from build123d import *

# Parameters (mm, degrees)
SKETCH1_R           = 2.15
SKETCH1_R_2         = 0.875
BOSS_EXTRUDE1_DEPTH = 12
SKETCH2_R           = 3
SKETCH2_R_2         = 0.874277104
BOSS_EXTRUDE2_DEPTH = 6.75
CUT_EXTRUDE1_DEPTH  = 14.5


with BuildPart() as part:
    # Sketch1 → Boss-Extrude1 (new body)
    with BuildSketch(Plane.XY):
        Circle(SKETCH1_R)
        Circle(SKETCH1_R_2, mode=Mode.SUBTRACT)
    extrude(amount=BOSS_EXTRUDE1_DEPTH)

    # Sketch2 → Boss-Extrude2 (add)
    with BuildSketch(Plane.XY.offset(12)):
        Circle(SKETCH2_R)
        Circle(SKETCH2_R_2, mode=Mode.SUBTRACT)
    extrude(amount=BOSS_EXTRUDE2_DEPTH)

    # Sketch3 → Cut-Revolve1 (revolve, cut)
    with BuildSketch(Plane(origin=(0, 0, 0), x_dir=(1, 0, 0), z_dir=(0, 1, 0))):
        Polygon((2.15, -12), (3, -13.75), (4.254862661, -13.125400589), (3.126580546, -11.371696522), align=None)
        Polygon((2.375, -18.75), (3, -15), (5.751760011, -16.421813113), (4.254862661, -20.939605223), align=None)
    revolve(axis=Axis((0, 0, 0), (0, 0, 1)), mode=Mode.SUBTRACT)

    # Sketch4 → Cut-Extrude1 (cut)
    with BuildSketch(Plane.XY.offset(18.75)):
        Polygon((0, 3.340763125), (-0.25, 3.340763125), (-0.25, 0.464842209), (0.25, 0.464842209), (0.25, 3.340763125), align=None)
        Polygon((3.340763125, 0), (3.340763125, 0.25), (0.464842209, 0.25), (0.464842209, -0.25), (3.340763125, -0.25), align=None)
        Polygon((0, -3.340763125), (0.25, -3.340763125), (0.25, -0.464842209), (-0.25, -0.464842209), (-0.25, -3.340763125), align=None)
        Polygon((-3.340763125, 0), (-3.340763125, -0.25), (-0.464842209, -0.25), (-0.464842209, 0.25), (-3.340763125, 0.25), align=None)
    extrude(amount=-CUT_EXTRUDE1_DEPTH, mode=Mode.SUBTRACT)


solid = part.part
Source: CAD feature listing. Evaluate the final solid. Frame: model axes, mm. A direction names the side the tool comes from. Round coordinates to 2 decimals unless told otherwise and drop trailing zeros. Loops run counter-clockwise (first coordinate to the right, second up) from the corner with the lowest first, then second, coordinate; pieces in that order, holes last. Notation, with made-up numbers: M 66,25 L 101,25 A19 cw 101,62 Z; hole C 0.25,9 d11. An arc over 180 degrees is marked long. Return JSON: item names as keys, results as strings. Group by question number.
1. Section query B-B on z = 14.25. Output: boundary loops of the cut face in (x, y).
2. Section query D-D on z = 3.5. Output: boundary loops of the cut face in (x, y) (3 decimals), and give its area (3 significant figures).
3. Reachability of faces 5 (the face through (1.7, 0.25, 11.6)), 6 (the face through (1.986, -0.823, 5.916)), 7 (the face through (-0.25, -1.7, 11.6)) from +Z, -Z, +X, -X, +Y, -Y: full face, straight path, thin tool, end or side. Return the list, or none.
4. Section query A-A on x = 0. Output: boundary loops of the cut face in (y, z) (3 decimals), and give its area (3 significant figures).
5. Mould query, pull axis Y, two halves, no side actions, for faces 1 (the face through (0.4, -0.78, 5.92)), 2 (the face through (1.84, 1.81, 12.89)), 3 (the face through (1.81, -1.84, 12.89)), 4 (the face through (1.7, -0.25, 11.6)). Classes: released by +Y, released by -Y, zero draft, split by the parting line, or undercut.
6. Pin query (flat end, axial travel): pin 1 (2.5 mm diameter, centred on x = 0, y = 0, fed in from -Z); pin 2 (1.1 mm diameter, centred on x = 2, z = 12, fed in from -Y); pin 3 (1.7 mm diameter, centred on x = 2, z = 9, fed in from +Y); pin 4 (1 mm diameter, centred on y = 1.5, z = 16, fed in from -X). Return the tip coordinate at first contact, or that it passes through.
7. Material intervals for line 1 along Y through (x, z) = (0, 2.75) (3 decimals); line 2 along X through (y, z) = (0.45, 9), sorted ascending. Write a range as from..to.
Checks:
{
 "1": {"outline": "M -2.99,-0.25 A3 ccw -0.25,-2.99 L -0.25,-0.84 A0.87 cw -0.84,-0.25 Z; M -2.99,0.25 L -0.84,0.25 A0.87 cw -0.25,0.84 L -0.25,2.99 A3 ccw Z; M 0.25,-2.99 A3 ccw 2.99,-0.25 L 0.84,-0.25 A0.87 cw 0.25,-0.84 Z; M 0.25,0.84 A0.87 cw 0.84,0.25 L 2.99,0.25 A3 ccw 0.25,2.99 Z"},
 "2": {"outline": "C 0,0 d4.3; hole C 0,0 d1.75", "area": "12.1 mm²"},
 "3": {"face 5": "+Z, +X, -X", "face 6": "-Z", "face 7": "+Z, +Y, -Y"},
 "4": {"outline": "M -2.15,0 L -0.875,0 L -0.875,4.25 L -2.15,4.25 Z; M 0.875,0 L 2.15,0 L 2.15,4.25 L 0.875,4.25 Z", "area": "10.8 mm²"},
 "5": {"face 1": "undercut", "face 2": "released by +Y", "face 3": "released by -Y", "face 4": "undercut"},
 "6": {"pin 1": "stops at z = 0", "pin 2": "stops at y = -1.7", "pin 3": "stops at y = 1.82", "pin 4": "stops at x = -2.67"},
 "7": {"line 1": "y = -2.15..-0.875, 0.875..2.15", "line 2": "x = -2.1..-0.75, 0.75..2.1"}
}
